Here's how the part is built. I have some questions about the finished solid (model axes, mm). Face numbers are marked on the shaded views. A direction names the side the tool comes from. Give positions to 0.01 mm unless a question says otherwise; leave off trailing zeros. Loops run counter-clockwise (first coordinate to the right, second up) from the corner with the lowest first, then second, coordinate; pieces in that order, holes last. Notation, with made-up numbers: M 57,-23 L 92,-23 A20 cw 92,-17 Z; hole C 1,-37.5 d1. An arc over 180 degrees is marked long. Answer as CSV lines item,"result". Start each with the question number.
Item 1: I want a section at D-D on z = -50.7. List the corners of the cut face in (x, y) for me.
Item 2: I want a section at C-C on z = -63.5. List the corners of the cut face in (x, y) for me, plus the area to 3 significant figures.
Item 3: For the marked faces 1 and 2, which set-ups out of +Z, -Z, +X, -X, +Y, -Y let a thin tool reach every point of the face, with its end or its side?
Item 4: If I drill on line 1 along Z through (x, y) = (0, 0.3); line 2 along Z through (x, y) = (-3.25, 1.5); line 3 along Y through (x, z) = (0, -71.5), over which ranges is the centre line in solid material (lowest first)? Write a range as from..to.
Item 5: I want a section at A-A on y = 0. List the corners of the cut face in (x, z) for me, plus the area to 3 significant figures.
Item 6: I want a section at B-B on x = 0. List the corners of the cut face in (y, z) for me, plus the area to 3 significant figures.
Item 7: Will these pins go through, and if not, where does the flat tip stop? P1, Ø1, axis at x = 1.5, z = -74.5, coming from the +Y side; P2, Ø1.5, axis at x = -3.5, z = -53, coming from the -Y side; P3, Ø2, axis at x = 0.5, z = -73, coming from the +Y side; P4, Ø1, axis at y = 2.5, z = -67, coming from the -X side.
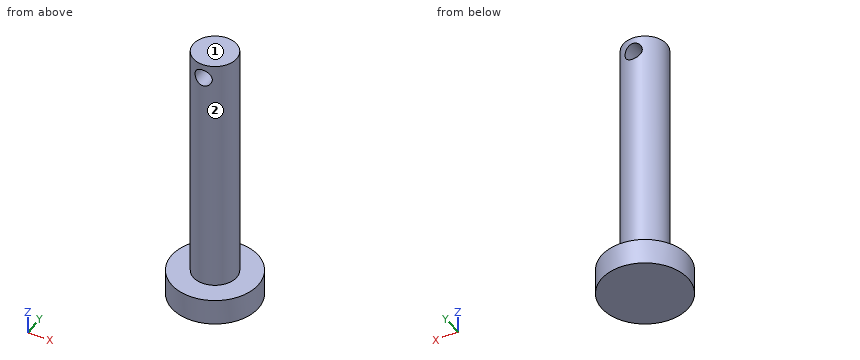
from build123d import *

# Parameters (mm, degrees)
CUT_EXTRUDE1_DEPTH      = 81.311892021
CUT_EXTRUDE1_DEPTH_BACK = 81.311892021
SKETCH3_W               = 130
SKETCH3_H               = 11.269282723
CUT_EXTRUDE2_DEPTH      = 81.311892021
CUT_EXTRUDE2_DEPTH_BACK = 81.311892021
SKETCH4_R               = 1


with BuildPart() as part:
    # Sketch2 → Revolve1 (revolve)
    with BuildSketch(Plane(origin=(0, 0, 0), x_dir=(0, 0, -1), z_dir=(1, 0, 0)), mode=Mode.PRIVATE) as revolve1_sk:
        Polygon((80, 0), (80, 5), (77, 5), (77, 2.5), (-80, 2.5), (-80, 0), align=None)
    revolve(revolve1_sk.sketch.rotate(Axis((0, 0, 80), (0, 0, -1)), 90), axis=Axis((0, 0, 80), (0, 0, -1)))

    # Sketch3 → Cut-Extrude1 (cut, two sides: drawn at the far end of the back side and taken through both)
    with BuildSketch(Plane(origin=(0, 0, 0), x_dir=(0, 0, -1), z_dir=(1, 0, 0)).offset(-CUT_EXTRUDE1_DEPTH_BACK)):
        with Locations((-16, 0.112241111)):
            Rectangle(SKETCH3_W, SKETCH3_H)
    extrude(amount=CUT_EXTRUDE1_DEPTH + CUT_EXTRUDE1_DEPTH_BACK, mode=Mode.SUBTRACT)

    # Sketch4 → Cut-Extrude2 (cut, two sides: drawn at the far end of the back side and taken through both)
    with BuildSketch(Plane(origin=(0, 0, 0), x_dir=(1, 0, 0), z_dir=(0, 1, 0)).offset(-CUT_EXTRUDE2_DEPTH_BACK)):
        with Locations(Location((0, 50.7, 0), (0, 0, 270))):
            Circle(SKETCH4_R)
    extrude(amount=CUT_EXTRUDE2_DEPTH + CUT_EXTRUDE2_DEPTH_BACK, mode=Mode.SUBTRACT)


solid = part.part
Result:
1,outline,"M -1,-2.29 L -1,2.29 A2.5 ccw Z; M 1,-2.29 A2.5 ccw 1,2.29 Z"
2,outline,"C 0,0 d5"
2,area,"19.6 mm^2"
3,face 1,"+Z, +X, -X, +Y, -Y"
3,face 2,"+Z"
4,line 1,"-80..-51.7, -49.7..-49"
4,line 2,"-80..-77"
4,line 3,"-2.5..2.5"
5,outline,"M -5,-80 L 5,-80 L 5,-77 L 2.5,-77 L 2.5,-49 L -2.5,-49 L -2.5,-77 L -5,-77 Z; hole C 0,-50.7 d2"
5,area,"167 mm^2"
6,outline,"M -5,-80 L 5,-80 L 5,-77 L 2.5,-77 L 2.5,-51.7 L -2.5,-51.7 L -2.5,-77 L -5,-77 Z; M -2.5,-49.7 L 2.5,-49.7 L 2.5,-49 L -2.5,-49 Z"
6,area,"160 mm^2"
7,P1,"y = 2.29"
7,P2,"through"
7,P3,"y = 2.5"
7,P4,"x = -1.5"
